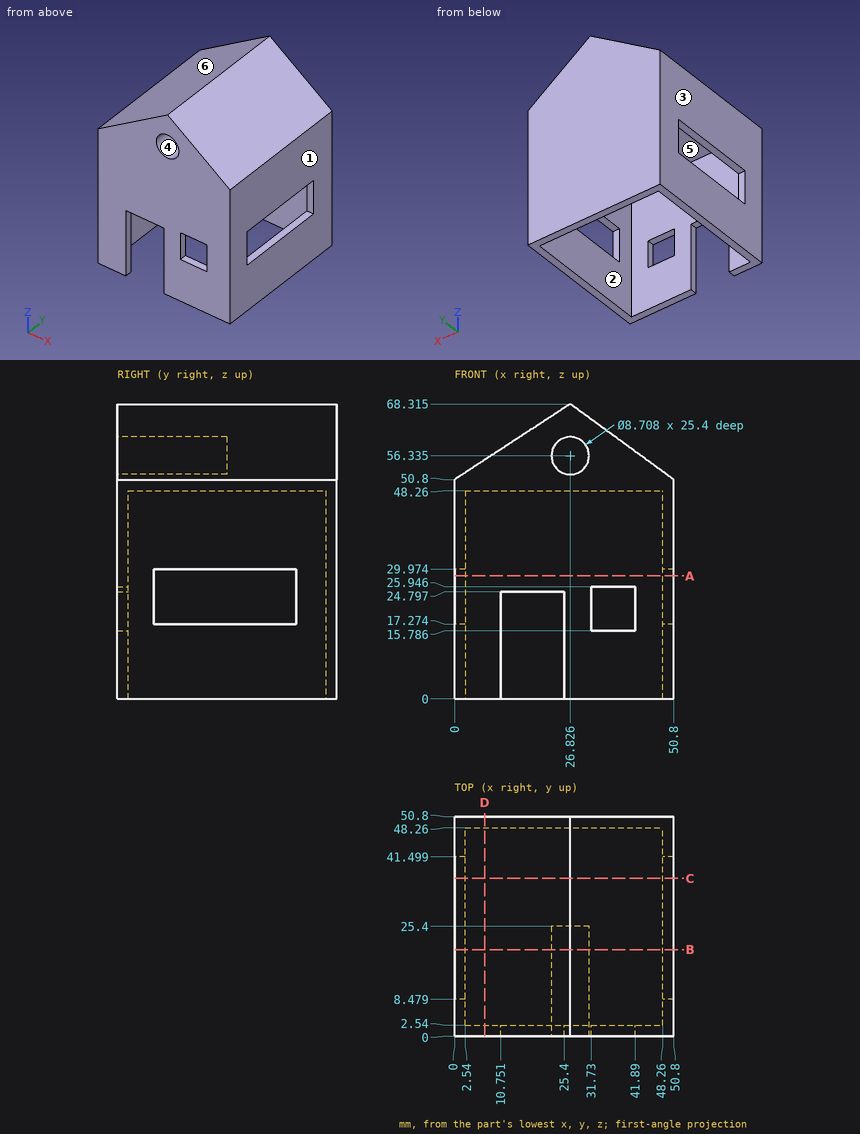
Could you check a few things on this drawing? It's one solid part, dimensions in mm from its lowest x, y, z. A direction names the side the tool comes from. Coordinates: 2 decimals unless noted, no trailing zeros. Order: outer loops, then holes, each group sorted by start corner. A loop starts at its lowest first (then second) coordinate and runs counter-clockwise, first axis right, second up.
1) We'd pull the mould along Z, two halves only. Please class the marked faces 3, 4, 5 and 6: +Z half, -Z half, draft (parallel to the pull), parting line (faces both ways), or undercut.
2) Imagine slicing it at A-A on z = 28.5. List the corners of the cut face in (x, y) for me.
3) I need wall thicknesses on line 1 (Y direction, x = 38.5, z = 38.5); line 2 (Y direction, x = 26, z = 58). Which ranges of each line are inside material? Lowest first, please.
4) Imagine slicing it at D-D on x = 7. List the corners of the cut face in (y, z) for me.
5) Imagine slicing it at B-B on y = 20. List the corners of the cut face in (x, z) for me (1 decimal), and give its area (3 significant figures).
6) Imagine slicing it at C-C on y = 36.5. List the corners of the cut face in (x, z) for me (1 decimal).
7) Which directions (+Z, -Z, +X, -X, +Y, -Y) give clear straight access to the entire face, cutting with the end or side of a thin tool? Please do the marked faces 1 and 2.
8) Will these pins go through, and if not, where does the flat tip stop? pin 1 (10 mm diameter, centred on x = 10.5, y = 42, fed in from +Z); pin 2 (0.8 mm diameter, centred on x = 37, y = 1.5, fed in from +Z) (1 decimal); pin 3 (12 mm diameter, centred on x = 21, y = 38, fed in from -Z).
Response values:
1. face 3: draft
1. face 4: undercut
1. face 5: -Z half
1. face 6: +Z half
2. outline: (0, 0) - (50.8, 0) - (50.8, 8.48) - (48.26, 8.48) - (48.26, 2.54) - (2.54, 2.54) - (2.54, 8.48) - (0, 8.48) - close; (0, 41.5) - (2.54, 41.5) - (2.54, 48.26) - (48.26, 48.26) - (48.26, 41.5) - (50.8, 41.5) - (50.8, 50.8) - (0, 50.8) - close
3. line 1: y = 0 to 2.54, 48.26 to 50.8
3. line 2: y = 25.4 to 50.8
4. outline: (0, 0) - (2.54, 0) - (2.54, 48.26) - (48.26, 48.26) - (48.26, 0) - (50.8, 0) - (50.8, 55.37) - (0, 55.37) - close
5. outline: (0, 0) - (2.5, 0) - (2.5, 17.3) - (0, 17.3) - close; (0, 30) - (2.5, 30) - (2.5, 48.3) - (48.3, 48.3) - (48.3, 30) - (50.8, 30) - (50.8, 50.8) - (26.8, 68.3) - (0, 50.8) - close; (48.3, 0) - (50.8, 0) - (50.8, 17.3) - (48.3, 17.3) - close; hole circle Ø8.7 at (26.8, 56.3)
5. area: 695 mm2
6. outline: (0, 0) - (2.5, 0) - (2.5, 17.3) - (0, 17.3) - close; (0, 30) - (2.5, 30) - (2.5, 48.3) - (48.3, 48.3) - (48.3, 30) - (50.8, 30) - (50.8, 50.8) - (26.8, 68.3) - (0, 50.8) - close; (48.3, 0) - (50.8, 0) - (50.8, 17.3) - (48.3, 17.3) - close
7. face 1: +Z, -Z, +X, +Y, -Y
7. face 2: -Z
8. pin 1: stops at z = 60.92
8. pin 2: stops at z = 61.2
8. pin 3: stops at z = 48.26
